from build123d import *

# Parameters (mm, degrees)
SKETCH007_R     = 39
PAD002_DEPTH    = 2
SKETCH005_R     = 3.2
POCKET003_DEPTH = 2
CHAMFER001_SIZE = 0.25


with BuildPart() as part:
    # Sketch007 → Pad002 (new body)
    with BuildSketch(Plane.XY):
        Circle(SKETCH007_R)
    extrude(amount=PAD002_DEPTH)

    # Sketch005 → Pocket003 (cut)
    with BuildSketch(Plane.XY):
        Circle(SKETCH005_R)
    extrude(amount=POCKET003_DEPTH, mode=Mode.SUBTRACT)

    # Chamfer001
    chamfer001_edges = [part.edges().sort_by_distance(p)[0] for p in [
        (-3.2, 0, 2),
        (-3.2, 0, 0),
    ]]
    chamfer(chamfer001_edges, length=CHAMFER001_SIZE)


solid = part.part
Geometry: final body of the model. Coordinates: model frame, mm. Round coordinates to 2 decimals unless told otherwise and drop trailing zeros. Order: outer loops, then holes, each group sorted by start corner. A loop starts at its lowest first (then second) coordinate and runs counter-clockwise, first axis right, second up. Notation, with made-up numbers: (8, -17) -> (40, -17) arc R19 cw to (40, 3) -> close; hole circle Ø8 at (61, 9). An arc over 180 degrees is marked (long way). Put each result on its own line as item: value. Start each with the question number.
Q1. Pull-direction query (Y, two-part tool) for faces 1 (the cylindrical face through (-2.539, -1.947, 0.99)), 2 (the flat face through (-1, -8, 2)), 3 (the cylindrical face through (-5.077, 38.668, 0.986)); classes: +Y half, -Y half, draft (parallel to the pull), parting line (faces both ways), or undercut.
Q2. Section D-D on x = -21.5. Return the cut outline in (y, z).
Q3. Section C-C on z = 1.1. Return the cut outline in (x, y).
Q4. Line query: probe 1 along Y at (x, z) = (0, 0.9); probe 2 along Y at (x, z) = (-22.5, 1.9); probe 3 along Y at (x, z) = (31.5, 0.5). Output: solid intervals per line, ascending.
Q5. First-contact query: pin 1 (1 mm diameter, centred on x = -5, z = 0, fed in from +Y). Flat tip, straight axial feed; report the tip coordinate or a pass-through.
Q6. Section A-A on x = 0. Return the cut outline in (y, z), and give its area (3 significant figures).
Ans:
1. face 1: undercut
1. face 2: draft
1. face 3: parting line
2. outline: (-32.54, 0) -> (32.54, 0) -> (32.54, 2) -> (-32.54, 2) -> close
3. outline: circle Ø78 at (0, 0); hole circle Ø6.4 at (0, 0)
4. probe 1: y = -39 to -3.2, 3.2 to 39
4. probe 2: y = -31.86 to 31.86
4. probe 3: y = -22.99 to 22.99
5. pin 1: stops at y = 38.74
6. outline: (-39, 0) -> (-3.45, 0) -> (-3.2, 0.25) -> (-3.2, 1.75) -> (-3.45, 2) -> (-39, 2) -> close; (3.2, 0.25) -> (3.45, 0) -> (39, 0) -> (39, 2) -> (3.45, 2) -> (3.2, 1.75) -> close
6. area: 143 mm2
